For this review, take the finished solid that the model builds, in its own axes (mm). Face numbers are marked on the shaded views. A direction names the side the tool comes from. Round coordinates to 2 decimals unless told otherwise and drop trailing zeros. Loops run counter-clockwise (first coordinate to the right, second up) from the corner with the lowest first, then second, coordinate; pieces in that order, holes last.
1. Consider section C-C on x = 72.5. State the section outline as (y, z) points, then the cut area to 3 significant figures.
2. To check wall thickness, follow line 1 along Z through (x, y) = (46, -0.5); line 2 along Z through (x, y) = (37, -17); line 3 along X through (y, z) = (24, -6). State the ranges of each line that lie inside material, in increasing order.
3. Tool access review of the marked faces 1 and 2: name each direction out of +Z, -Z, +X, -X, +Y, -Y from which nothing blocks a thin tool from reaching the whole face with its end or side.
4. Draft analysis for pull direction Z (two halves, no side actions). For the marked faces 3, 4, 5 and 6, state which applies: released by +Z, released by -Z, zero draft, split by the parting line, or undercut.
5. Consider section A-A on y = 30. State the section outline as (x, z) points, then the cut area to 3 significant figures.
6. Consider section D-D on x = 31.5. State how many separate pieces and enclosed holes the cut face has, then the cut area to 3 significant figures.
7. Clearance check with flat-ended pins moving along their axes: pin 1 Ø6.5 at (y, z) = (42, -67) entering from +X; pin 2 Ø5.5 at (x, z) = (82, -48) entering from +Y; pin 3 Ø12 at (y, z) = (36, -19) entering from +X; pin 4 Ø10 at (x, y) = (43.5, -16.5) entering from +Z. State where each tip first meets the part, or that it passes through.
8. Consider section B-B on z = -36.5. State the section outline as (x, y) points, then the cut area to 3 significant figures.
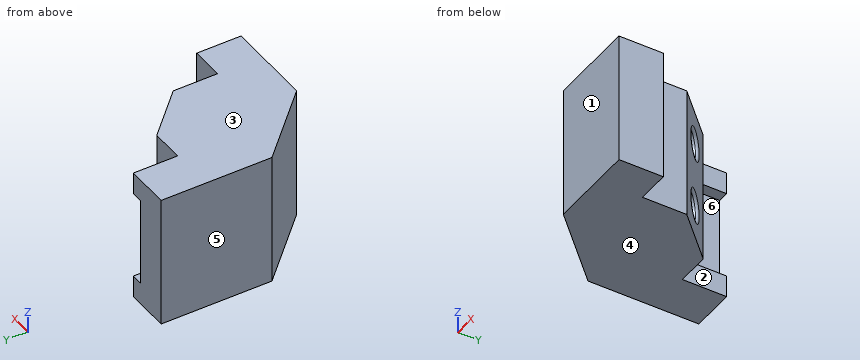
from build123d import *

# Parameters (mm, degrees)
BOSS_EXTRUDE2_DEPTH = 76.2
SKETCH3_W           = 6.35
SKETCH3_H           = 50.8
CUT_EXTRUDE1_DEPTH  = 25.4
SKETCH4_R           = 7.62
CUT_EXTRUDE2_DEPTH  = 53.34
FILLET2_R           = 1.524


with BuildPart() as part:
    # Sketch2 → Boss-Extrude2 (new body)
    with BuildSketch(Plane.XY):
        Polygon((0, 48.351318045), (0, -15.148681955), (38.1, -53.248681955), (88.9, -53.248681955), (88.9, -27.848681955), (69.85, -27.848681955), (69.85, -2.448681955), (44.45, 22.951318045), (25.4, 22.951318045), (25.4, 48.351318045), align=None)
    extrude(amount=-BOSS_EXTRUDE2_DEPTH)

    # Sketch3 → Cut-Extrude1 (cut)
    with BuildSketch(Plane(origin=(0, 48.351318045, 0), x_dir=(1, 0, 0), z_dir=(0, 1, 0))):
        with Locations((22.225, 38.1)):
            Rectangle(SKETCH3_W, SKETCH3_H)
    extrude(amount=-CUT_EXTRUDE1_DEPTH, mode=Mode.SUBTRACT)

    # Sketch4 → Cut-Extrude2 (cut)
    with BuildSketch(Plane(origin=(33.700659023, 33.700659023, 0), x_dir=(0, 0, -1), z_dir=(0.7071067811865488, 0.7071067811865462, 0))):
        with Locations(Location((19.05, -33.165088281, 0), (0, 0, 90))):
            Circle(SKETCH4_R)
        with Locations(Location((57.15, -33.165088281, 0), (0, 0, 90))):
            Circle(SKETCH4_R)
    extrude(amount=-CUT_EXTRUDE2_DEPTH, mode=Mode.SUBTRACT)

    # Fillet2
    fillet2_edges = [part.edges().sort_by_distance(p)[0] for p in [
        (62.540071517, 4.861246528, -19.05),
        (62.540071517, 4.861246528, -57.15),
    ]]
    fillet(fillet2_edges, radius=FILLET2_R)


solid = part.part
Resolved:
1. outline: (-53.25, -76.2) - (-27.85, -76.2) - (-27.85, 0) - (-53.25, 0) - close
1. area: 1,940 mm2
2. line 1: z = -76.2 to -64.76, -49.54 to -26.66, -11.44 to 0
2. line 2: z = -76.2 to -62.88, -51.42 to -24.78, -13.32 to 0
2. line 3: x = 0 to 25.4
3. face 1: +Z, -Z, +X, -X, -Y
3. face 2: +Z, -Z, +X, +Y
4. face 3: released by +Z
4. face 4: released by -Z
4. face 5: zero draft
4. face 6: undercut
5. outline: (0, -76.2) - (25.4, -76.2) - (25.4, -63.5) - (19.05, -63.5) - (19.05, -12.7) - (25.4, -12.7) - (25.4, 0) - (0, 0) - close
5. area: 1,610 mm2
6. separate pieces: 1
6. enclosed holes: 2
6. area: 4,790 mm2
7. pin 1: stops at x = 25.4
7. pin 2: stops at y = -27.85
7. pin 3: stops at x = 19.05
7. pin 4: stops at z = 0
8. outline: (0, -15.15) - (38.1, -53.25) - (88.9, -53.25) - (88.9, -27.85) - (69.85, -27.85) - (69.85, -2.45) - (44.45, 22.95) - (19.05, 22.95) - (19.05, 48.35) - (0, 48.35) - close
8. area: 5,240 mm2
